For this review, take the finished solid that the model builds, in its own axes (mm). A direction names the side the tool comes from. Round coordinates to 2 decimals unless told otherwise and drop trailing zeros. Write each loop counter-clockwise with the first axis right and the second up, starting at its lowest first coordinate (ties: lowest second). Pieces come first, ordered by that corner, then holes. Notation, with made-up numbers: M 83,-39 L 92,-39 A24 ccw 92,-8 Z; hole C -22,-28.5 d6. An arc over 180 degrees is marked long. Write each question's results on one line, items separated by ' | '. Start each with the question number.
Autodesk Inventor part; units mm, degrees
ref_plane "YZ Plane" through (0, 0, 0) normal (1, 0, 0) x (0, 1, 0)
ref_plane "XZ Plane" through (0, 0, 0) normal (0, 1, 0) x (-1, 0, 0)
ref_plane "XY Plane" through (0, 0, 0) normal (0, 0, 1) x (1, 0, 0)
sketch "Sketch1" plane through (0, 0, 0) normal (0, 1, 0) x (-1, 0, 0)
  line L0 (18, 30.25) -> (-18, 30.25) construction
  line L1 (-18, 30.25) -> (-18, -32.75) construction
  line L2 (-18, -32.75) -> (18, -32.75) construction
  line L3 (18, -32.75) -> (18, 30.25) construction
  line L4 (11, 30.25) -> (-11, 30.25)
  line L5 (11, 30.25) -> (11, 23.25)
  line L6 (11, 23.25) -> (18, 23.25)
  line L7 (14.75, -32.75) -> (-14.75, -32.75)
  line L8 (14.75, -32.75) -> (14.75, -23.25)
  line L9 (14.75, -23.25) -> (18, -23.25)
  line L10 (14.75, 0) -> (18, 0)
  line L11 (-11, 30.25) -> (-11, 23.25)
  line L12 (-11, 23.25) -> (-18, 23.25)
  line L13 (-14.75, -32.75) -> (-14.75, -23.25)
  line L14 (-14.75, -23.25) -> (-18, -23.25)
  line L15 (18, 23.25) -> (18, -23.25)
  line L16 (-18, -23.25) -> (-18, 23.25)
  point P0 (0, 0)
  point P1 (0, 30.25)
  point P2 (0, -32.75)
  point P3 (-18, -6.9939)
  point P4 (18, 0)
  dimension "d0" = 36
  dimension "d1" = 63
  dimension "d2" = 22
  dimension "d3" = 7
  dimension "d4" = 29.5
  dimension "d5" = 9.5
  dimension "d10" = 7
  dimension "d11" = 9.5
extrude "Extrusion1" add sketch "Sketch1" along normal blind 1.57
chamfer "Chamfer2" distance 1 angle 45 4 edges at (11, 0.785, 30.25) (-11, 0.785, 30.25) (14.75, 0.785, -32.75) (-14.75, 0.785, -32.75)
sketch "Sketch2" plane through (0, 1.57, 0) normal (0, 1, 0) x (1, 0, 0)
  line L0 (-18, -23.25) -> (-11, -23.25)
  line L1 (-18, 23.25) -> (-18, -23.25)
  point P0 (0, 0)
  point P1 (15, -21)
  point P2 (15, 21)
  point P3 (-15, -21)
  point P4 (-15, 21)
  dimension "d20" = 42
  dimension "d21" = 42
  dimension "d22" = 30
  dimension "d28" = 2.25
  dimension "d36" = 3
hole "Hole1" at (15, 1.57, 21) at (15, 1.57, -21) at (-15, 1.57, 21) at (-15, 1.57, -21) direction (0, -1, 0) diameter 2.2 end through all
sketch "Sketch3" plane through (0, 1.57, 0) normal (0, 1, 0) x (1, 0, 0)
  line L0 (-18, 1.5) -> (-14.75, 1.5)
  line L1 (-14.75, 1.5) -> (-14.75, 6.5)
  line L2 (-14.75, 6.5) -> (-18, 6.5)
  line L3 (-18, 23.25) -> (-18, -23.25)
  circle A0 centre (-15, 21) radius 1.1
  line L4 (0, 0) -> (0, 8.9759) construction
  line L5 (18, 1.5) -> (14.75, 1.5)
  line L6 (14.75, 1.5) -> (14.75, 6.5)
  line L7 (14.75, 6.5) -> (18, 6.5)
  line L8 (18, 23.25) -> (18, -21.75)
  point P0 (-18, -21.75)
  point P1 (-14.75, 4)
  dimension "d37" = 5
  dimension "d38" = 3.25
  dimension "d39" = 3.25
  dimension "d40" = 17
extrude "Extrusion2" cut sketch "Sketch3" against normal through all contours L3 L2 L1 L0 | L5 L6 L7 L8
chamfer "Chamfer3" distance 1.5 angle 45 6 edges at (-18, 0.785, 23.25) (18, 0.785, 23.25) (18, 0.785, -1.5) (18, 0.785, -6.5) (-18, 0.785, -1.5) (-18, 0.785, -6.5)
equation "\"d39\" = d38"
properties part number "LFRboard"
Item 1: Insertion check: P1, Ø0.5, axis at x = 16, y = 1, coming from the -Z side; P2, Ø0.5, axis at y = 0.5, z = -28, coming from the -X side; P3, Ø0.8, axis at y = 1, z = 27, coming from the -X side. Each pin has a flat end and moves straight along its axis. Give the tip position at first contact, or say it passes through.
Item 2: For faces 1 (the flat face through (-11, 1, 26)), 2 (the flat face through (-14.75, 1, -4)), 3 (the flat face through (-14.75, 1, -28)), list the 3-axis set-ups (+Z, -Z, +X, -X, +Y, -Y) from which the entire face can be reached by the end or side of a thin tool; tool diameter is ignored.
Item 3: We need section B-B on y = 1.25. State how many separate pieces and enclosed holes the cut face has, then the cut area to 3 significant figures.
Item 4: We need section A-A on z = 21. State the section outline as (x, y) points.
Item 5: For probe 1 along X at (y, z) = (1.1, 21); probe 2 along Z at (x, y) = (-15, 0.75); probe 3 along X at (y, z) = (1.05, -22), list the stretches that pass through material, from the lowest coordinate up.
Item 6: Mouldability with a two-part tool opening along X and no side actions: class faces 4 (the flat face through (0, 0, -1)), 5 (the cylindrical face through (15.67, 0.77, 20.13)), 6 (the flat face through (11, 1, 26)) as pulls with the +X half, pulls with the -X half, needs draft (parallel to the pull), parting line crosses it, or undercut.
Numbers:
1) P1: stops at z = -23.25 | P2: stops at x = -14.75 | P3: stops at x = -11
2) face 1: +Z, -X, +Y, -Y | face 2: -X, +Y, -Y | face 3: -Z, -X, +Y, -Y
3) separate pieces: 1 | enclosed holes: 4 | area: 2,050 mm^2
4) outline: M -18,0 L -16.1,0 L -16.1,1.57 L -18,1.57 Z; M -13.9,0 L 13.9,0 L 13.9,1.57 L -13.9,1.57 Z; M 16.1,0 L 18,0 L 18,1.57 L 16.1,1.57 Z
5) probe 1: x = -18 to -16.1, -13.9 to 13.9, 16.1 to 18 | probe 2: z = -23.25 to -22.1, -19.9 to -6.5, -1.5 to 19.9, 22.1 to 23.25 | probe 3: x = -18 to -15.46, -14.54 to 14.54, 15.46 to 18
6) face 4: needs draft | face 5: undercut | face 6: pulls with the +X half
